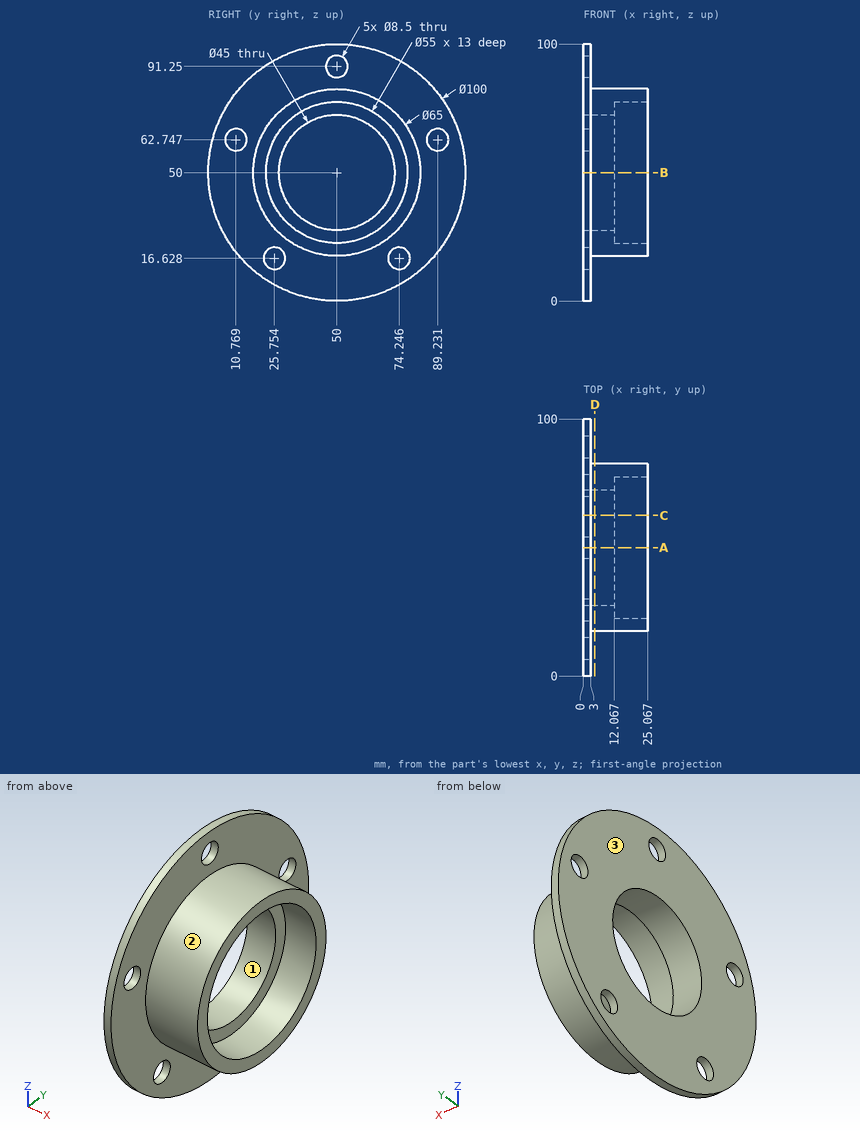
Input: dimensioned drawing with shaded views. Units: mm. Origin: part minimum x, y, z. Coordinates: 2 decimals unless noted, no trailing zeros. Order: outer loops, then holes, each group sorted by start corner. A loop starts at its lowest first (then second) coordinate and runs counter-clockwise, first axis right, second up.
(1) Section query B-B (z = 50). Return the cut outline in (x, y), plus the area to 3 significant figures.
(2) Section query A-A (y = 50). Return the cut outline in (x, z), plus the area to 3 significant figures.
(3) Section query D-D (x = 4.5). Return the cut outline in (y, z).
(4) Material intervals for probe 1 along Y at (x, z) = (8.5, 50); probe 2 along Y at (x, z) = (15.75, 50); probe 3 along X at (y, z) = (70.5, 66.5), sorted ascending.
(5) Section query C-C (y = 62.5). Return the cut outline in (x, z) (1 decimal).
(6) First-contact query: pin 1 (2 mm diameter, centred on x = 8.5, y = 69.5, fed in from -Z); pin 2 (1 mm diameter, centred on x = 12, y = 76.5, fed in from +Z); pin 3 (13.5 mm diameter, centred on y = 74.25, z = 16.63, fed in from +X). Flat tips, straight axial feed; report the tip coordinate or a pass-through.
(7) Draft query along Z for the marked faces 1, 2 and 3. Return one class per face: pulls with the +Z half, pulls with the -Z half, needs draft (parallel to the pull), parting line crosses it, or undercut.
Solution:
1. outline: (0, 0) - (3, 0) - (3, 17.5) - (25.07, 17.5) - (25.07, 22.5) - (12.07, 22.5) - (12.07, 27.5) - (0, 27.5) - close; (0, 72.5) - (12.07, 72.5) - (12.07, 77.5) - (25.07, 77.5) - (25.07, 82.5) - (3, 82.5) - (3, 100) - (0, 100) - close
1. area: 476 mm2
2. outline: (0, 0) - (3, 0) - (3, 17.5) - (25.07, 17.5) - (25.07, 22.5) - (12.07, 22.5) - (12.07, 27.5) - (0, 27.5) - close; (0, 72.5) - (12.07, 72.5) - (12.07, 77.5) - (25.07, 77.5) - (25.07, 82.5) - (3, 82.5) - (3, 87) - (0, 87) - close; (0, 95.5) - (3, 95.5) - (3, 100) - (0, 100) - close
2. area: 451 mm2
3. outline: circle Ø65 at (50, 50); hole circle Ø45 at (50, 50)
4. probe 1: y = 17.5 to 27.5, 72.5 to 82.5
4. probe 2: y = 17.5 to 22.5, 77.5 to 82.5
4. probe 3: x = 0 to 12.07
5. outline: (0, 1.6) - (3, 1.6) - (3, 20) - (25.1, 20) - (25.1, 25.5) - (12.1, 25.5) - (12.1, 31.3) - (0, 31.3) - close; (0, 68.7) - (12.1, 68.7) - (12.1, 74.5) - (25.1, 74.5) - (25.1, 80) - (3, 80) - (3, 98.4) - (0, 98.4) - close
6. pin 1: stops at z = 23.28
6. pin 2: stops at z = 69.5
6. pin 3: stops at x = 3
7. face 1: undercut
7. face 2: parting line crosses it
7. face 3: needs draft
